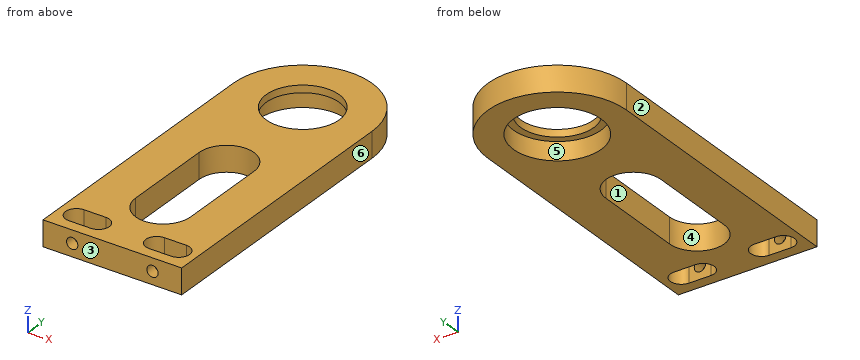
from build123d import *

# Parameters (mm, degrees)
SKETCH_1_R         = 10
SKETCH_1_R_2       = 19
EXTRUDE_1_DEPTH    = 7
SKETCH2_R          = 12.025
CUT_EXTRUDE2_DEPTH = 5
SKETCH3_R          = 1.55
CUT_EXTRUDE3_DEPTH = 5


with BuildPart() as part:
    # 草图1 → 凸台-拉伸1 (new body)
    # profile 1 of 3: a face of its own
    with BuildSketch(Plane.XY):
        with BuildLine():
            ThreePointArc((19, 75), (0, 94), (-19, 75))
            ThreePointArc((-19, 75), (0, 56), (19, 75))
        make_face()
        with Locations((0, 75)):
            Circle(SKETCH_1_R, mode=Mode.SUBTRACT)
    # profile 2 of 3: a face of its own
    with BuildSketch(Plane.XY):
        with BuildLine():
            Line((-19, 7), (-19, 0))
            Line((-19, 0), (19, 0))
            Line((19, 0), (19, 7))
            Line((19, 7), (19, 75))
            ThreePointArc((19, 75), (0, 56), (-19, 75))
            Line((-19, 75), (-19, 7))
        make_face()
        with BuildLine():
            ThreePointArc((-8, 9), (-5, 6), (-8, 3))
            Line((-8, 3), (-14, 3))
            ThreePointArc((-14, 3), (-17, 6), (-14, 9))
            Line((-14, 9), (-8, 9))
        make_face(mode=Mode.SUBTRACT)
        with BuildLine():
            Line((14, 3), (8, 3))
            ThreePointArc((8, 3), (5, 6), (8, 9))
            Line((8, 9), (14, 9))
            ThreePointArc((14, 9), (17, 6), (14, 3))
        make_face(mode=Mode.SUBTRACT)
        with BuildLine():
            ThreePointArc((-7.5, 45), (0, 52.5), (7.5, 45))
            Line((7.5, 45), (7.5, 20))
            ThreePointArc((7.5, 20), (0, 12.5), (-7.5, 20))
            Line((-7.5, 20), (-7.5, 45))
        make_face(mode=Mode.SUBTRACT)
    # profile 3 of 3: a face of its own
    with BuildSketch(Plane.XY):
        with Locations((0, 75)):
            Circle(SKETCH_1_R_2)
        with Locations((0, 75)):
            Circle(SKETCH_1_R, mode=Mode.SUBTRACT)
    extrude(amount=EXTRUDE_1_DEPTH)

    # Sketch2 → Cut-Extrude2 (cut)
    with BuildSketch(Plane(origin=(0, 0, 0), x_dir=(-1, 0, 0), z_dir=(0, 0, -1))):
        with Locations((0, 75)):
            Circle(SKETCH2_R)
    extrude(amount=-CUT_EXTRUDE2_DEPTH, mode=Mode.SUBTRACT)

    # Sketch3 → Cut-Extrude3 (cut)
    with BuildSketch(Plane.XZ):
        with Locations(Location((11, 3.5, 0), (0, 0, 270))):
            Circle(SKETCH3_R)
        with Locations((-11, 3.5)):
            Circle(SKETCH3_R)
    extrude(amount=-CUT_EXTRUDE3_DEPTH, mode=Mode.SUBTRACT)


solid = part.part
Model file for the job. Use its own axes, mm. Face numbers are marked on the shaded views. A direction names the side the tool comes from. Coordinates: 2 decimals unless noted, no trailing zeros. Write each loop counter-clockwise with the first axis right and the second up, starting at its lowest first coordinate (ties: lowest second). Pieces come first, ordered by that corner, then holes. Notation, with made-up numbers: (38.5, -18) -> (65.5, -18) arc R25 cw to (65.5, 14) -> close; hole circle Ø1 at (23.5, 36.25). An arc over 180 degrees is marked (long way). One line per item, written item: value. Start each with the question number.
1) Slice it at B-B on y = 33. Write the cut outline in (x, z), then the cut area to 3 significant figures.
2) Flat gauge pins, fed straight in: pin 1 Ø3 at (x, z) = (-7, 3) entering from +Y; pin 2 Ø16 at (x, y) = (0, 75) entering from +Z; pin 3 Ø3.5 at (x, z) = (11, 3.5) entering from +Y; pin 4 Ø1.5 at (x, z) = (13.5, 2.5) entering from +Y. Where does each tip first touch, or does it go through?
3) Slice it at C-C on x = 11. Write the cut outline in (y, z).
4) Slice it at A-A on y = 6. Write the cut outline in (x, z), then the cut area to 3 significant figures.
5) Which spindle directions (+Z, -Z, +X, -X, +Y, -Y) get a long thin tool onto all of the face, cutting with end or side? Do the marked faces 1 and 2. Say none if no direction does.
6) Probe probe 1 along Y at (x, z) = (0, 3.95) (3 decimals); probe 2 along X at (y, z) = (75, 6.3); probe 3 along X at (y, z) = (30.5, 2). List the from-to ranges inside material, lowest first.
7) Pull direction Y, two halves, no side cores. Call the marked faces 3, 4, 5 and 6: +Y half, -Y half, draft (parallel to the pull), parting line (faces both ways), or undercut.
Answers follow:
1. outline: (-19, 0) -> (-7.5, 0) -> (-7.5, 7) -> (-19, 7) -> close; (7.5, 0) -> (19, 0) -> (19, 7) -> (7.5, 7) -> close
1. area: 161 mm2
2. pin 1: y = 93.19
2. pin 2: through
2. pin 3: y = 91.6
2. pin 4: y = 89.09
3. outline: (0, 0) -> (3, 0) -> (3, 1.95) -> (0, 1.95) -> close; (0, 5.05) -> (3, 5.05) -> (3, 7) -> (0, 7) -> close; (9, 0) -> (70.14, 0) -> (70.14, 5) -> (79.86, 5) -> (79.86, 0) -> (90.49, 0) -> (90.49, 7) -> (9, 7) -> close
4. outline: (-19, 0) -> (-17, 0) -> (-17, 7) -> (-19, 7) -> close; (-5, 0) -> (5, 0) -> (5, 7) -> (-5, 7) -> close; (17, 0) -> (19, 0) -> (19, 7) -> (17, 7) -> close
4. area: 98.0 mm2
5. face 1: +Z, -Z
5. face 2: +Z, -Z, -X, +Y, -Y
6. probe 1: 0 to 12.5, 52.5 to 62.975, 87.025 to 94
6. probe 2: -19 to -10, 10 to 19
6. probe 3: -19 to -7.5, 7.5 to 19
7. face 3: -Y half
7. face 4: undercut
7. face 5: undercut
7. face 6: draft
